```python
from build123d import *

# Parameters (mm, degrees)
SKETCH_1_W          = 145
SKETCH_1_H          = 272.434969596
EXTRUDE_1_DEPTH     = 10
SKETCH_2_W          = 58
SKETCH_2_H          = 150
SKETCH_2_W_2        = 12.5
SKETCH_2_H_2        = 100
CUT_EXTRUDE_1_DEPTH = 10
FILLET_1_R          = 15
FILLET_2_R          = 3


with BuildPart() as part:
    # 草图1 → 凸台-拉伸1 (new body)
    with BuildSketch(Plane.XY):
        Rectangle(SKETCH_1_W, SKETCH_1_H)
    extrude(amount=EXTRUDE_1_DEPTH)

    # 草图2 → 切除-拉伸1 (cut)
    with BuildSketch(Plane.XY):
        with Locations((-43.5, 61.217484798)):
            Rectangle(SKETCH_2_W, SKETCH_2_H)
        Polygon((-72.5, -98.782515202), (-72.5, -136.217484798), (-42.5, -136.217484798), align=None)
        with Locations((30.25, 6.217484798)):
            Rectangle(SKETCH_2_W_2, SKETCH_2_H_2)
    extrude(amount=CUT_EXTRUDE_1_DEPTH, mode=Mode.SUBTRACT)

    # 圆角1
    fillet_1_edges = [part.edges().sort_by_distance(p)[0] for p in [
        (-72.5, -13.782515202, 5),
    ]]
    fillet(fillet_1_edges, radius=FILLET_1_R)

    # 圆角2
    fillet_2_edges = [part.edges().sort_by_distance(p)[0] for p in [
        (36.5, -43.782515202, 5),
        (36.5, 56.217484798, 5),
        (24, 56.217484798, 5),
        (24, -43.782515202, 5),
    ]]
    fillet(fillet_2_edges, radius=FILLET_2_R)


solid = part.part
```
Here's how the part is built. I have some questions about the finished solid (model axes, mm). A direction names the side the tool comes from. Round coordinates to 2 decimals unless told otherwise and drop trailing zeros. Loops run counter-clockwise (first coordinate to the right, second up) from the corner with the lowest first, then second, coordinate; pieces in that order, holes last.
1. Will these pins go through, and if not, where does the flat tip stop? pin 1 (5 mm diameter, centred on x = -39.5, z = 7, fed in from +Y); pin 2 (1.5 mm diameter, centred on y = 69.5, z = 9, fed in from -X); pin 3 (4 mm diameter, centred on x = -55, z = 3, fed in from -Y).
Answers:
pin 1: stops at y = -13.78
pin 2: stops at x = -14.5
pin 3: stops at y = -123.12
2. Suppose I cut it at D-D, the plane x = -27. Please give me the cut outline in (y, z), and give its area (3 significant figures).
Answers:
outline: (-136.22, 0) - (-13.78, 0) - (-13.78, 10) - (-136.22, 10) - close
area: 1,220 mm2
3. Suppose I cut it at B-B, the plane z = 7.25. Please give me the cut outline in (x, y), and give its area (3 significant figures).
Answers:
outline: (-72.5, -98.78) - (-42.5, -136.22) - (72.5, -136.22) - (72.5, 136.22) - (-14.5, 136.22) - (-14.5, -13.78) - (-57.5, -13.78) arc R15 ccw to (-72.5, -28.78) - close; hole (24, -40.78) arc R3 ccw to (27, -43.78) - (33.5, -43.78) arc R3 ccw to (36.5, -40.78) - (36.5, 53.22) arc R3 ccw to (33.5, 56.22) - (27, 56.22) arc R3 ccw to (24, 53.22) - close
area: 29,000 mm2
4. Suppose I cut it at A-A, the plane y = -34.5. Please give me the cut outline in (x, z).
Answers:
outline: (-72.5, 0) - (24, 0) - (24, 10) - (-72.5, 10) - close; (36.5, 0) - (72.5, 0) - (72.5, 10) - (36.5, 10) - close
5. Suppose I cut it at C-C, the plane y = 31.5. Please give me the cut outline in (x, z), and give its area (3 significant figures).
Answers:
outline: (-14.5, 0) - (24, 0) - (24, 10) - (-14.5, 10) - close; (36.5, 0) - (72.5, 0) - (72.5, 10) - (36.5, 10) - close
area: 745 mm2
6. For faces 4 (the face through (36.5, 6, 5)), 5 (the face through (14, -136.217, 5)), 6 (the face through (-14.5, 60, 5)), which set-ups out of +Z, -Z, +X, -X, +Y, -Y let a thin tool reach every point of the face, with its end or its side?
Answers:
face 4: +Z, -Z
face 5: +Z, -Z, +X, -X, -Y
face 6: +Z, -Z, -X, +Y
7. Thinking about a two-plate mould opening in X: for faces 1 (the face through (24, 6, 5)), 2 (the face through (-57.29, -117.76, 4.93)), 3 (the face through (15, -28, 10)), which applies, released by +X, released by -X, zero draft, split by the parting line, or undercut?
Answers:
face 1: undercut
face 2: released by -X
face 3: zero draft
8. If I drill on probe 1 along X at (y, z) = (-41, 2.75); probe 2 along X at (y, z) = (17.5, 9.5); probe 3 along X at (y, z) = (88, 1.5), over which ranges is the centre line in solid material (lowest first)?
Answers:
probe 1: x = -72.5 to 24.01, 36.49 to 72.5
probe 2: x = -14.5 to 24, 36.5 to 72.5
probe 3: x = -14.5 to 72.5
